Read the model definition and answer for the solid it produces. Units are mm, in the model's axes. A direction names the side the tool comes from. Coordinates: 2 decimals unless noted, no trailing zeros. Write each loop counter-clockwise with the first axis right and the second up, starting at its lowest first coordinate (ties: lowest second). Pieces come first, ordered by that corner, then holes. Notation, with made-up numbers: (70.25, 24.5) -> (79.25, 24.5) arc R13 cw to (79.25, 31.5) -> close; hole circle Ø9 at (76, 45). An arc over 180 degrees is marked (long way). Answer in a Markdown table with one row per item. Add a question column.
Item 1: Which of the six approach directions +Z, -Z, +X, -X, +Y, -Y give full straight-line access (tool end or side, diameter ignored) to faces 1 (the face through (8, -58, 1.905)), 2 (the face through (10.873, -56, -8)), 3 (the face through (10.873, -56, 8)), 4 (the face through (1.827, -56, -13))?
Item 2: Straight lines are drawn through the part: line 1 (Y direction, x = -7, z = 0) (3 decimals); line 2 (X direction, y = -50.25, z = 0); line 3 (X direction, y = -19, z = -0.5). For each, find the intervals that lie inside material, in ascending order. Write a range as from..to.
Item 3: Given pin 1 Ø1 at (y, z) = (17.5, 5.5) entering from -X; pin 2 Ø5 at (y, z) = (-41.5, 5.5) entering from -X; pin 3 Ø4.5 at (x, z) = (6, -9.5) entering from -Y, each flat-ended and moving along its own axis, determine where each tip first touches the part or whether it passes through.
Item 4: Section D-D on x = 6.35 is taken. Write down the section's boundary in (y, z) (3 decimals), then the cut area to 3 significant figures.
Item 5: Section A-A on y = -55.88 is taken. Count the separate pieces of the cut face and the enclosed holes in it, then the cut area to 3 significant figures.
Item 6: Section B-B on x = 0 is taken. Write down the section's boundary in (y, z), then the cut area to 3 significant figures.
Item 7: Section C-C on z = 9 is taken. Write down the section's boundary in (x, y).
Item 8: For a pull along Y with two mould halves and no side action, classify faces 5 (the face through (2.004, -56, 0)), 6 (the face through (10, -59.69, 0)), 7 (the face through (-14, 44, -2.921)) as +Y half, -Y half, draft (parallel to the pull), parting line (faces both ways), or undercut.
```python
from build123d import *

# Parameters (mm, degrees)
SKETCH1_R               = 19.05
BOSS_EXTRUDE1_DEPTH     = 50.8
SKETCH2_R               = 14.82725
BOSS_EXTRUDE2_DEPTH     = 8.89
CUT_EXTRUDE2_DEPTH      = 114.727064061
CUT_EXTRUDE2_DEPTH_BACK = 95.25
SKETCH4_R               = 16.51
CUT_EXTRUDE3_REACH      = 115.727
SKETCH5_R               = 12.28725
BOSS_EXTRUDE3_START     = -16.51
SKETCH8_W               = 12.7
SKETCH8_H               = 12.7
BOSS_EXTRUDE3_DEPTH     = 12.065
CUT_EXTRUDE5_DEPTH      = 66.488175269
CUT_EXTRUDE5_DEPTH_BACK = 66.488175269
SKETCH9_W               = 9.046009644
SKETCH9_H               = 7.62
SKETCH10_W              = 12.7
SKETCH10_H              = 3.81
BOSS_EXTRUDE4_DEPTH     = 7.62
CUT_EXTRUDE6_DEPTH      = 67.067470248
CUT_EXTRUDE6_DEPTH_BACK = 67.067470248
SKETCH11_R              = 2.4
SKETCH12_R              = 1.2
CUT_EXTRUDE7_DEPTH      = 67.916467517
CUT_EXTRUDE8_DEPTH      = 15.845


with BuildPart() as part:
    # Sketch1 → Boss-Extrude1 (new, symmetric)
    with BuildSketch(Plane(origin=(0, 0, 0), x_dir=(1, 0, 0), z_dir=(0, 1, 0))):
        with Locations(Location((0, 0, 0), (0, 0, 270))):
            Circle(SKETCH1_R)
    extrude(amount=BOSS_EXTRUDE1_DEPTH, both=True)

    # Sketch2 → Boss-Extrude2 (add)
    with BuildSketch(Plane.XZ.offset(50.8)):
        with Locations(Location((0, 0, 0), (0, 0, 270))):
            Circle(SKETCH2_R)
    extrude(amount=BOSS_EXTRUDE2_DEPTH)

    # Sketch4 → Cut-Extrude2 (cut, two sides: drawn at the far end of the back side and taken through both)
    with BuildSketch(Plane(origin=(0, 50.8, 0), x_dir=(1, 0, 0), z_dir=(0, 1, 0)).offset(-CUT_EXTRUDE2_DEPTH_BACK)):
        with Locations(Location((0, 0, 0), (0, 0, 270))):
            Circle(SKETCH4_R)
    extrude(amount=CUT_EXTRUDE2_DEPTH + CUT_EXTRUDE2_DEPTH_BACK, mode=Mode.SUBTRACT)

    # Sketch5 → Cut-Extrude3 (cut, up to next)
    with BuildSketch(Plane.XZ.offset(59.69), mode=Mode.PRIVATE) as cut_extrude3_sk1:
        with Locations(Location((0, 0, 0), (0, 0, 270))):
            Circle(SKETCH5_R)
    cut_extrude3_tool1 = extrude(cut_extrude3_sk1.sketch, amount=-CUT_EXTRUDE3_REACH, mode=Mode.PRIVATE) & part.part
    add(cut_extrude3_tool1.solids().sort_by_distance((0, -59.69, 0))[0], mode=Mode.SUBTRACT)

    # Sketch8 → Boss-Extrude3 (add)
    with BuildSketch(Plane(origin=(0, 0, 0), x_dir=(0, 0, -1), z_dir=(1, 0, 0)).offset(BOSS_EXTRUDE3_START)):
        with Locations((0, 44.45)):
            Rectangle(SKETCH8_W, SKETCH8_H)
    extrude(amount=BOSS_EXTRUDE3_DEPTH)

    # Sketch9 → Cut-Extrude5 (cut, two sides: drawn at the far end of the back side and taken through both)
    with BuildSketch(Plane.XY.offset(-CUT_EXTRUDE5_DEPTH_BACK)):
        with Locations((6.35, -55.88)):
            Rectangle(SKETCH9_W, SKETCH9_H)
    extrude(amount=CUT_EXTRUDE5_DEPTH + CUT_EXTRUDE5_DEPTH_BACK, mode=Mode.SUBTRACT)

    # Sketch10 → Boss-Extrude4 (add)
    with BuildSketch(Plane.XZ.offset(59.69)):
        with Locations((8.354363895, 0)):
            Rectangle(SKETCH10_W, SKETCH10_H)
    extrude(amount=-BOSS_EXTRUDE4_DEPTH)

    # Sketch11 → Cut-Extrude6 (cut, two sides: drawn at the far end of the back side and taken through both)
    with BuildSketch(Plane.XY.offset(1.905).offset(-CUT_EXTRUDE6_DEPTH_BACK)):
        with Locations((6.35, -55.88)):
            Circle(SKETCH11_R)
    extrude(amount=CUT_EXTRUDE6_DEPTH + CUT_EXTRUDE6_DEPTH_BACK, mode=Mode.SUBTRACT)

    # Sketch12 → Cut-Extrude7 (cut, through all)
    with BuildSketch(Plane(origin=(-4.445, 0, 0), x_dir=(0, 0, -1), z_dir=(1, 0, 0))):
        with Locations((0, 41.275)):
            Circle(SKETCH12_R)
        with Locations((0, 47.625)):
            Circle(SKETCH12_R)
    extrude(amount=-CUT_EXTRUDE7_DEPTH, mode=Mode.SUBTRACT)

    # Sketch14 → Cut-Extrude8 (cut)
    with BuildSketch(Plane.ZY.offset(25.4)):
        with BuildLine():
            Line((-2.921, 41.275), (-2.921, 47.625))
            ThreePointArc((-2.921, 47.625), (0, 50.546), (2.921, 47.625))
            Line((2.921, 47.625), (2.921, 41.275))
            ThreePointArc((2.921, 41.275), (0, 38.354), (-2.921, 41.275))
        make_face()
    extrude(amount=-CUT_EXTRUDE8_DEPTH, mode=Mode.SUBTRACT)


solid = part.part
```
Results below:
| question | item | result |
|---|---|---|
| 1 | face 1 | +Y, -Y |
| 1 | face 2 | -Z, -Y |
| 1 | face 3 | +Z, -Y |
| 1 | face 4 | +Z, -Z, +X, -Y |
| 2 | line 1 | y = 38.1..40.075, 42.475..46.425, 48.825..50.8 |
| 2 | line 2 | x = -19.05..-12.29, 12.29..19.05 |
| 2 | line 3 | x = -19.04..-16.5, 16.5..19.04 |
| 3 | pin 1 | stops at x = -18.38 |
| 3 | pin 2 | stops at x = -18.81 |
| 3 | pin 3 | stops at y = -52.07 |
| 4 | outline | (-59.69, -1.905) -> (-58.28, -1.905) -> (-58.28, 1.905) -> (-59.69, 1.905) -> close; (-53.48, -1.905) -> (-52.07, -1.905) -> (-52.07, 1.905) -> (-53.48, 1.905) -> close; (-52.07, -13.399) -> (-50.8, -13.399) -> (-50.8, -17.961) -> (50.8, -17.961) -> (50.8, -15.24) -> (-44.45, -15.24) -> (-44.45, -10.519) -> (-52.07, -10.519) -> close; (-52.07, 10.519) -> (-44.45, 10.519) -> (-44.45, 15.24) -> (50.8, 15.24) -> (50.8, 17.961) -> (-50.8, 17.961) -> (-50.8, 13.399) -> (-52.07, 13.399) -> close |
| 4 | area | 631 mm2 |
| 5 | separate pieces | 3 |
| 5 | enclosed holes | 0 |
| 5 | area | 182 mm2 |
| 6 | outline | (-59.69, -14.83) -> (-50.8, -14.83) -> (-50.8, -19.05) -> (50.8, -19.05) -> (50.8, -16.51) -> (-44.45, -16.51) -> (-44.45, -12.29) -> (-59.69, -12.29) -> close; (-59.69, 12.29) -> (-44.45, 12.29) -> (-44.45, 16.51) -> (50.8, 16.51) -> (50.8, 19.05) -> (-50.8, 19.05) -> (-50.8, 14.83) -> (-59.69, 14.83) -> close |
| 6 | area | 615 mm2 |
| 7 | outline | (-16.79, -50.8) -> (-11.78, -50.8) -> (-11.78, -59.69) -> (-8.37, -59.69) -> (-8.37, -44.45) -> (-13.84, -44.45) -> (-13.84, 50.8) -> (-16.79, 50.8) -> close; (8.37, -52.07) -> (10.87, -52.07) -> (10.87, -59.69) -> (11.78, -59.69) -> (11.78, -50.8) -> (16.79, -50.8) -> (16.79, 50.8) -> (13.84, 50.8) -> (13.84, -44.45) -> (8.37, -44.45) -> close |
| 8 | face 5 | draft |
| 8 | face 6 | -Y half |
| 8 | face 7 | undercut |
